Design review of the part built by this model. Coordinates are the model's own, in mm. Coordinates: 2 decimals unless noted, no trailing zeros. Loops run counter-clockwise (first coordinate to the right, second up) from the corner with the lowest first, then second, coordinate; pieces in that order, holes last. Notation, with made-up numbers: (-15.75, 48) -> (5.25, 48) arc R9 cw to (5.25, 63) -> close; hole circle Ø10 at (-19, -27.75). An arc over 180 degrees is marked (long way). Use a Markdown table: item, result. Add a question column.
Q1. For probe 1 along X at (y, z) = (110, 4.5); probe 2 along X at (y, z) = (92, 0.5); probe 3 along Z at (x, y) = (-11.5, 408), list the stretches that pass through material, from the lowest coordinate up.
Q2. Clearance check with flat-ended pins moving along their axes: pin 1 Ø0.8 at (y, z) = (435, 0.5) entering from +X; pin 2 Ø1.5 at (x, z) = (7.5, 3.5) entering from +Y; pin 3 Ø1.1 at (y, z) = (288.5, 0.5) entering from -X; pin 4 Ø1.5 at (x, y) = (10, 412) entering from +Z. State where each tip first meets the part, or that it passes through.
Q3. Take a section at A-A on z = 4. Write out the cut boundary in (x, y).
from build123d import *

# Parameters (mm, degrees)
RAIL_DEPTH       = 469
SLOTS_DEPTH      = 470.386301462
SLOTS_DEPTH_BACK = 470.386301462


with BuildPart() as part:
    # Sketch1 → Rail (new body)
    with BuildSketch(Plane(origin=(0, 0, 0), x_dir=(1, 0, 0), z_dir=(0, 1, 0))):
        Polygon((-13.5, 0), (13.5, 0), (13.5, -6.5), (17.5, -6.5), (17.5, -7.5), (12.5, -7.5), (12.5, -1), (-12.5, -1), (-12.5, -7.5), (-17.5, -7.5), (-17.5, -6.5), (-13.5, -6.5), align=None)
    extrude(amount=RAIL_DEPTH)

    # Sketch2 → Slots (cut, two sides: drawn at the far end of the back side and taken through both)
    with BuildSketch(Plane.XY.offset(-SLOTS_DEPTH_BACK)):
        with BuildLine():
            Line((-2.6, 7.6), (-2.6, 17.4))
            ThreePointArc((-2.6, 17.4), (0, 20), (2.6, 17.4))
            Line((2.6, 17.4), (2.6, 7.6))
            ThreePointArc((2.6, 7.6), (0, 5), (-2.6, 7.6))
        make_face()
        with BuildLine():
            Line((-2.6, 32.6), (-2.6, 42.4))
            ThreePointArc((-2.6, 42.4), (0, 45), (2.6, 42.4))
            Line((2.6, 42.4), (2.6, 32.6))
            ThreePointArc((2.6, 32.6), (0, 30), (-2.6, 32.6))
        make_face()
        with BuildLine():
            Line((-2.6, 57.6), (-2.6, 67.4))
            ThreePointArc((-2.6, 67.4), (0, 70), (2.6, 67.4))
            Line((2.6, 67.4), (2.6, 57.6))
            ThreePointArc((2.6, 57.6), (0, 55), (-2.6, 57.6))
        make_face()
        with BuildLine():
            Line((-2.6, 82.6), (-2.6, 92.4))
            ThreePointArc((-2.6, 92.4), (0, 95), (2.6, 92.4))
            Line((2.6, 92.4), (2.6, 82.6))
            ThreePointArc((2.6, 82.6), (0, 80), (-2.6, 82.6))
        make_face()
        with BuildLine():
            Line((-2.6, 107.6), (-2.6, 117.4))
            ThreePointArc((-2.6, 117.4), (0, 120), (2.6, 117.4))
            Line((2.6, 117.4), (2.6, 107.6))
            ThreePointArc((2.6, 107.6), (0, 105), (-2.6, 107.6))
        make_face()
        with BuildLine():
            Line((-2.6, 132.6), (-2.6, 142.4))
            ThreePointArc((-2.6, 142.4), (0, 145), (2.6, 142.4))
            Line((2.6, 142.4), (2.6, 132.6))
            ThreePointArc((2.6, 132.6), (0, 130), (-2.6, 132.6))
        make_face()
        with BuildLine():
            Line((-2.6, 157.6), (-2.6, 167.4))
            ThreePointArc((-2.6, 167.4), (0, 170), (2.6, 167.4))
            Line((2.6, 167.4), (2.6, 157.6))
            ThreePointArc((2.6, 157.6), (0, 155), (-2.6, 157.6))
        make_face()
        with BuildLine():
            Line((-2.6, 182.6), (-2.6, 192.4))
            ThreePointArc((-2.6, 192.4), (0, 195), (2.6, 192.4))
            Line((2.6, 192.4), (2.6, 182.6))
            ThreePointArc((2.6, 182.6), (0, 180), (-2.6, 182.6))
        make_face()
        with BuildLine():
            Line((-2.6, 207.6), (-2.6, 217.4))
            ThreePointArc((-2.6, 217.4), (0, 220), (2.6, 217.4))
            Line((2.6, 217.4), (2.6, 207.6))
            ThreePointArc((2.6, 207.6), (0, 205), (-2.6, 207.6))
        make_face()
        with BuildLine():
            Line((-2.6, 232.6), (-2.6, 242.4))
            ThreePointArc((-2.6, 242.4), (0, 245), (2.6, 242.4))
            Line((2.6, 242.4), (2.6, 232.6))
            ThreePointArc((2.6, 232.6), (0, 230), (-2.6, 232.6))
        make_face()
        with BuildLine():
            Line((-2.6, 257.6), (-2.6, 267.4))
            ThreePointArc((-2.6, 267.4), (0, 270), (2.6, 267.4))
            Line((2.6, 267.4), (2.6, 257.6))
            ThreePointArc((2.6, 257.6), (0, 255), (-2.6, 257.6))
        make_face()
        with BuildLine():
            Line((-2.6, 282.6), (-2.6, 292.4))
            ThreePointArc((-2.6, 292.4), (0, 295), (2.6, 292.4))
            Line((2.6, 292.4), (2.6, 282.6))
            ThreePointArc((2.6, 282.6), (0, 280), (-2.6, 282.6))
        make_face()
        with BuildLine():
            Line((-2.6, 307.6), (-2.6, 317.4))
            ThreePointArc((-2.6, 317.4), (0, 320), (2.6, 317.4))
            Line((2.6, 317.4), (2.6, 307.6))
            ThreePointArc((2.6, 307.6), (0, 305), (-2.6, 307.6))
        make_face()
        with BuildLine():
            Line((-2.6, 332.6), (-2.6, 342.4))
            ThreePointArc((-2.6, 342.4), (0, 345), (2.6, 342.4))
            Line((2.6, 342.4), (2.6, 332.6))
            ThreePointArc((2.6, 332.6), (0, 330), (-2.6, 332.6))
        make_face()
        with BuildLine():
            Line((-2.6, 357.6), (-2.6, 367.4))
            ThreePointArc((-2.6, 367.4), (0, 370), (2.6, 367.4))
            Line((2.6, 367.4), (2.6, 357.6))
            ThreePointArc((2.6, 357.6), (0, 355), (-2.6, 357.6))
        make_face()
        with BuildLine():
            Line((-2.6, 382.6), (-2.6, 392.4))
            ThreePointArc((-2.6, 392.4), (0, 395), (2.6, 392.4))
            Line((2.6, 392.4), (2.6, 382.6))
            ThreePointArc((2.6, 382.6), (0, 380), (-2.6, 382.6))
        make_face()
        with BuildLine():
            Line((-2.6, 407.6), (-2.6, 417.4))
            ThreePointArc((-2.6, 417.4), (0, 420), (2.6, 417.4))
            Line((2.6, 417.4), (2.6, 407.6))
            ThreePointArc((2.6, 407.6), (0, 405), (-2.6, 407.6))
        make_face()
        with BuildLine():
            Line((-2.6, 432.6), (-2.6, 442.4))
            ThreePointArc((-2.6, 442.4), (0, 445), (2.6, 442.4))
            Line((2.6, 442.4), (2.6, 432.6))
            ThreePointArc((2.6, 432.6), (0, 430), (-2.6, 432.6))
        make_face()
    extrude(amount=SLOTS_DEPTH + SLOTS_DEPTH_BACK, mode=Mode.SUBTRACT)


solid = part.part
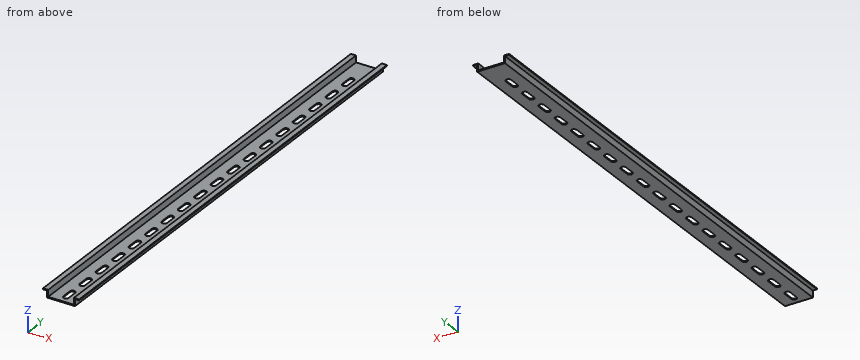
Answer list:
| question | item | result |
|---|---|---|
| 1 | probe 1 | -13.5 to -12.5, 12.5 to 13.5 |
| 1 | probe 2 | -13.5 to -2.6, 2.6 to 13.5 |
| 1 | probe 3 | 0 to 1 |
| 2 | pin 1 | x = 13.5 |
| 2 | pin 2 | through |
| 2 | pin 3 | x = -13.5 |
| 2 | pin 4 | z = 1 |
| 3 | outline | (-13.5, 0) -> (-12.5, 0) -> (-12.5, 469) -> (-13.5, 469) -> close; (12.5, 0) -> (13.5, 0) -> (13.5, 469) -> (12.5, 469) -> close |
